Verification items for the finished model (mm, model axes). A direction names the side the tool comes from. Give positions to 0.01 mm unless a question says otherwise; leave off trailing zeros. Order: outer loops, then holes, each group sorted by start corner. A loop starts at its lowest first (then second) coordinate and runs counter-clockwise, first axis right, second up. Notation, with made-up numbers: (-5.75, -16) -> (40.25, -16) arc R31 ccw to (40.25, 11) -> close; hole circle Ø5 at (46, -4.75). An arc over 180 degrees is marked (long way). Write each question's results on one line, items separated by ' | '. Start each with the question number.
1. Cross-section at B-B, the plane x = 157. Enter the section's corners in (y, z).
2. Cross-section at C-C, the plane z = 0.5. Enter the section's corners in (x, y), then the cut area to 3 significant figures.
3. Material ranges on L1, parallel to X at y = 1, z = 82 (3 decimals); L2, parallel to Y at x = 187, z = 29; L3, parallel to X at y = 1.5, z = 17.5, recorded low to high. Write a range as from..to.
4. Depth check by flat-ended pin: pin 1 Ø1.3 at (x, y) = (246.5, 2) entering from +Z; pin 2 Ø1.3 at (y, z) = (0.5, 57.5) entering from -X; pin 3 Ø0.5 at (x, y) = (231.5, -0.5) entering from -Z. Enter the tip coordinate at first touch or a pass-through.
5. Mould release check, pull along X, two halves, no side actions. Record for faces 1 (the face through (149.829, 1.252, 86.456)), 2 (the face through (193, 2.54, 47)), 3 (the face through (144.258, 1, 60)): +X half, -X half, draft (parallel to the pull), parting line (faces both ways), or undercut.
6. Cross-section at A-A, the plane y = -2. Enter the section's corners in (x, z).
7. Cross-section at D-D, the plane x = 217.5. Enter the section's corners in (y, z).
8. Set-up check for faces 4 (the face through (149.89, 1.25, -15.37)), 5 (the face through (231.15, 1.91, 28.91)), 6 (the face through (193, 1, 84.407)), 7 (the face through (144.258, 1, 10)), 8 (the face through (243.393, 1.288, 82.663)): record each of +Z, -Z, +X, -X, +Y, -Y from which the full face is reachable in a straight line by a thin tool's end or side.
from build123d import *

# Parameters (mm, degrees)
SKETCH1_R           = 4.1275
BOSS_EXTRUDE1_DEPTH = 2.54
SKETCH2_R           = 1.5
CUT_EXTRUDE1_DEPTH  = 267.081941915
CUT_EXTRUDE2_DEPTH  = 1.27
SKETCH1_5_W         = 30.48
SKETCH1_5_H         = 7.62
BOSS_EXTRUDE2_DEPTH = 3.556
FILLET1_R           = 2.54


with BuildPart() as part:
    # Sketch1 → Boss-Extrude1 (new body)
    with BuildSketch(Plane(origin=(0, 0, 0), x_dir=(1, 0, 0), z_dir=(0, 1, 0))):
        Polygon((239.739404703, 17.423809937), (235.698289449, 13.382694682), (151.878289449, 13.382694682), (147.837174194, 17.423809937), (140.217174194, 9.803809937), (144.258289449, 5.762694682), (144.258289449, -26.876305318), (136.638289449, -26.876305318), (136.638289449, -44.148305318), (144.258289449, -44.148305318), (144.258289449, -76.787305318), (140.217174194, -80.828420572), (147.837174194, -88.448420572), (151.878289449, -84.407305318), (235.698289449, -84.407305318), (239.739404703, -88.448420572), (247.359404703, -80.828420572), (243.318289449, -76.787305318), (243.318289449, -44.148305318), (250.938289449, -44.148305318), (250.938289449, -26.876305318), (243.318289449, -26.876305318), (243.318289449, 5.762694682), (247.359404703, 9.803809937), align=None)
        with Locations(Location((193.788289449, -35.512305318, 0), (0, 0, 270))):
            Circle(SKETCH1_R, mode=Mode.SUBTRACT)
    extrude(amount=BOSS_EXTRUDE1_DEPTH)

    # Sketch2 → Cut-Extrude1 (cut, through all)
    with BuildSketch(Plane(origin=(0, 2.54, 0), x_dir=(1, 0, 0), z_dir=(0, 1, 0))):
        with Locations(Location((145.448426066, 10.832301944, 0), (0, 0, 270))):
            Circle(SKETCH2_R)
        with Locations(Location((242.128152831, 10.832301944, 0), (0, 0, 270))):
            Circle(SKETCH2_R)
        with Locations(Location((242.128152831, -81.856912579, 0), (0, 0, 270))):
            Circle(SKETCH2_R)
        with Locations(Location((145.448426066, -81.856912579, 0), (0, 0, 270))):
            Circle(SKETCH2_R)
    extrude(amount=-CUT_EXTRUDE1_DEPTH, mode=Mode.SUBTRACT)

    # Sketch3 → Cut-Extrude2 (cut)
    with BuildSketch(Plane(origin=(0, 2.54, 0), x_dir=(1, 0, 0), z_dir=(0, 1, 0))):
        Polygon((150.442755261, -23.843216639), (160.890404833, -23.843216639), (160.890404833, -25.742789289), (152.104881329, -25.742789289), (152.104881329, -31.441507237), (160.890404833, -31.441507237), (160.890404833, -33.341079887), (152.104881329, -33.341079887), (152.104881329, -40.464477323), (160.890404833, -40.464477323), (160.890404833, -42.364049972), (150.442755261, -42.364049972), align=None)
        Polygon((164.21465697, -42.364049972), (164.21465697, -23.843216639), (164.563406636, -23.843216639), (176.799325773, -38.420210663), (176.799325773, -23.843216639), (178.461451842, -23.843216639), (178.461451842, -42.364049972), (178.083021353, -42.364049972), (165.876783038, -27.820446874), (165.876783038, -42.364049972), align=None)
        Polygon((206.100233893, -25.166133306), (207.753879726, -25.166133306), (213.486518615, -38.719138948), (219.219157504, -25.166133306), (220.872803338, -25.166133306), (213.596761671, -42.364049972), (213.37627556, -42.364049972), align=None)
        Polygon((222.636692226, -25.166133306), (224.404026211, -25.166133306), (228.923991489, -32.555863124), (233.437066575, -25.166133306), (235.20440056, -25.166133306), (229.692247782, -34.188838384), (229.692247782, -42.364049972), (228.148845004, -42.364049972), (228.148845004, -34.188838384), align=None)
    extrude(amount=-CUT_EXTRUDE2_DEPTH, mode=Mode.SUBTRACT)

    # Sketch1_5 → Boss-Extrude2 (add)
    with BuildSketch(Plane(origin=(0, 0, 0), x_dir=(1, 0, 0), z_dir=(0, 1, 0))):
        with Locations((159.498289449, -35.512305318)):
            Rectangle(SKETCH1_5_W, SKETCH1_5_H)
        with Locations((228.078289449, -35.512305318)):
            Rectangle(SKETCH1_5_W, SKETCH1_5_H)
    extrude(amount=-BOSS_EXTRUDE2_DEPTH)

    # Fillet1
    fillet1_edges = [part.edges().sort_by_distance(p)[0] for p in [
        (159.498289449, -3.556, 39.322305318),
        (159.498289449, -3.556, 31.702305318),
        (228.078289449, -3.556, 31.702305318),
        (228.078289449, -3.556, 39.322305318),
    ]]
    fillet(fillet1_edges, radius=FILLET1_R)


solid = part.part
Results below:
1) outline: (-3.56, 34.24) arc R2.54 ccw to (-1.02, 31.7) -> (0, 31.7) -> (0, -13.38) -> (2.54, -13.38) -> (2.54, 23.84) -> (1.27, 23.84) -> (1.27, 25.74) -> (2.54, 25.74) -> (2.54, 31.44) -> (1.27, 31.44) -> (1.27, 33.34) -> (2.54, 33.34) -> (2.54, 40.46) -> (1.27, 40.46) -> (1.27, 42.36) -> (2.54, 42.36) -> (2.54, 84.41) -> (0, 84.41) -> (0, 39.32) -> (-1.02, 39.32) arc R2.54 ccw to (-3.56, 36.78) -> close
2) outline: (144.26, 0) -> (243.32, 0) -> (243.32, 2.54) -> (144.26, 2.54) -> close | area: 252 mm²
3) L1: x = 141.389..143.955, 146.942..240.635, 243.621..246.188 | L2: y = 0..2.54 | L3: x = 144.26..243.32
4) pin 1: stops at z = 82.34 | pin 2: stops at x = 144.26 | pin 3: stops at z = 31.7
5) face 1: undercut | face 2: draft | face 3: -X half
6) outline: (144.26, 31.9) -> (174.74, 31.9) -> (174.74, 39.12) -> (144.26, 39.12) -> close; (212.84, 31.9) -> (243.32, 31.9) -> (243.32, 39.12) -> (212.84, 39.12) -> close
7) outline: (-3.56, 34.24) arc R2.54 ccw to (-1.02, 31.7) -> (0, 31.7) -> (0, -13.38) -> (2.54, -13.38) -> (2.54, 29.23) -> (1.27, 29.23) -> (1.27, 33.14) -> (2.54, 33.14) -> (2.54, 84.41) -> (0, 84.41) -> (0, 39.32) -> (-1.02, 39.32) arc R2.54 ccw to (-3.56, 36.78) -> close
8) face 4: -Z, +Y, -Y | face 5: +Y | face 6: +Z, +Y, -Y | face 7: -X, +Y, -Y | face 8: +Y, -Y
